Verification items for the finished model (mm, model axes). Face numbers are marked on the shaded views. A direction names the side the tool comes from. Round coordinates to 2 decimals unless told otherwise and drop trailing zeros. Order: outer loops, then holes, each group sorted by start corner. A loop starts at its lowest first (then second) coordinate and runs counter-clockwise, first axis right, second up. Notation, with made-up numbers: M 51.25,65.25 L 99.25,65.25 A28 ccw 99.25,88.25 Z; hole C 23,8.25 d6. An arc over 180 degrees is marked long. Use one line per item in the form item = value. Start each with the question number.
Item 1: Thickness scan on probe 1 along X at (y, z) = (16, -62.5); probe 2 along X at (y, z) = (217, -29); probe 3 along Y at (x, z) = (-22, 28.5). Record the ranges inside material, lowest first. Write a range as [from, to].
Item 2: Go/stop test with flat-tipped pins: pin 1 Ø10 at (x, y) = (88.5, 96.5) entering from +Z; pin 2 Ø4 at (x, y) = (170.5, -139) entering from +Z; pin 3 Ø2 at (x, y) = (211, -204) entering from +Z. Record where each tip stops, or that it passes through.
Item 3: Cross-section at A-A on y = -188. Enter the section's corners in (x, z), then the cut area to 3 significant figures.
Item 4: Tool access check on the marked faces 1 and 2. Record the directions out of +Z, -Z, +X, -X, +Y, -Y that give a thin tool (end or side, any length) a straight path to the whole face; none if there is none.
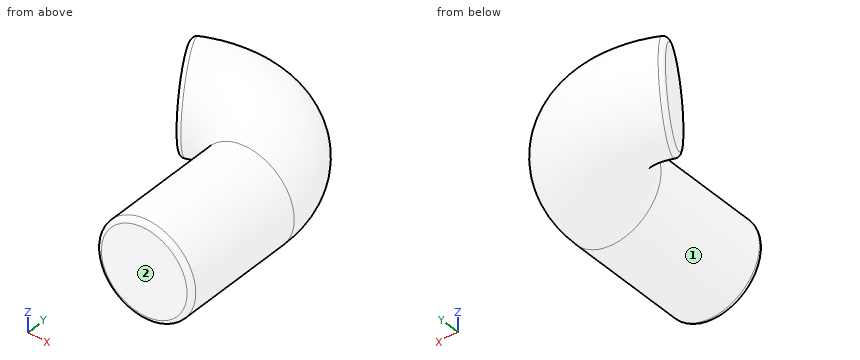
from build123d import *

# Parameters (mm, degrees)
F1_R      = 100
F2_FACE_R = 100
F4_R      = 158.537666862
F4_R_2    = 100
F5_DEPTH  = 261
F6_R      = 10
F7_R      = 10


with BuildPart() as f2:
    # F2: sweep along a path in F0
    with BuildLine(Plane.XY) as f2_path:
        ThreePointArc((161.8, 0), (80.7807923206, 140.1916673417), (-81.1382397041, 139.9850922696))
    # F1 (on Front) → F2 (sweep)
    with BuildSketch(Plane.XZ):
        with Locations((161.8, 0)):
            Circle(F1_R)
    sweep(path=f2_path.line)

    # F3: sweep along a path in F0
    with BuildLine(Plane.XY) as f3_path:
        Line((161.8, 0), (161.8, -261.8))
    # F2_face (on face) → F3 (sweep)
    with BuildSketch(Plane(origin=(161.8, 0, 0), x_dir=(1, 0, 0), z_dir=(0, -1, 0))):
        Circle(F2_FACE_R)
    sweep(path=f3_path.line)

    # F4 (on face) → F5 (cut)
    with BuildSketch(Plane.XZ.offset(261.8)):
        with Locations((161.8, 0)):
            Circle(F4_R)
        with Locations((161.8, 0)):
            Circle(F4_R_2, mode=Mode.SUBTRACT)
    extrude(amount=-F5_DEPTH, mode=Mode.SUBTRACT)

    # F6
    f6_edges = [f2.edges().sort_by_distance(p)[0] for p in [
        (61.8, 0, 0),
        (61.8, -261.8, 0),
        (261.8, -130.9, 0),
    ]]
    fillet(f6_edges, radius=F6_R)

    # F7
    f7_edges = [f2.edges().sort_by_distance(p)[0] for p in [
        (-30.990996, 53.46773, 0),
    ]]
    fillet(f7_edges, radius=F7_R)


solid = f2.part
Output values:
q1.probe_1 = [82.19, 239.33]
q1.probe_2 = [-125.06, 138.63]
q1.probe_3 = [62.17, 256.71]
q2.pin_1 = 96.6
q2.pin_2 = 99.78
q2.pin_3 = 87.62
q3.outline = C 161.8,0 d200
q3.area = 31,400 mm2
q4.face_1 = -Y
q4.face_2 = +Z, -Z, +X, -X, -Y
